Model file for the job. Use its own axes, mm. Coordinates: 2 decimals unless noted, no trailing zeros. Order: outer loops, then holes, each group sorted by start corner. A loop starts at its lowest first (then second) coordinate and runs counter-clockwise, first axis right, second up.
from build123d import *

# Parameters (mm, degrees)
SKETCH1_W           = 300
SKETCH1_H           = 400
SUPPORT_PLATE_DEPTH = 20
SKETCH2_R           = 6.5
BOLT_HOLES_DEPTH    = 21


with BuildPart() as part:
    # Sketch1 → Support Plate (new body)
    with BuildSketch(Plane(origin=(0, 0, 0), x_dir=(1, 0, 0), z_dir=(0, 1, 0))):
        Rectangle(SKETCH1_W, SKETCH1_H)
    extrude(amount=-SUPPORT_PLATE_DEPTH)

    # Sketch2 → Bolt Holes (cut, through all)
    with BuildSketch(Plane(origin=(0, 0, 0), x_dir=(-1, 0, 0), z_dir=(0, 1, 0))):
        with Locations((-100, -60)):
            Circle(SKETCH2_R)
        with Locations((50, -60)):
            Circle(SKETCH2_R)
        with Locations((50, 60)):
            Circle(SKETCH2_R)
        with Locations((-100, 60)):
            Circle(SKETCH2_R)
    extrude(amount=-BOLT_HOLES_DEPTH, mode=Mode.SUBTRACT)


solid = part.part
Q1. Probe line 1 (Z direction, x = -50, y = -7.75); line 2 (X direction, y = -9.25, z = 61.5); line 3 (Z direction, x = 97, y = -8.5). List the from-to ranges inside material, lowest first.
Established:
line 1: z = -200 to -66.5, -53.5 to 53.5, 66.5 to 200
line 2: x = -150 to -56.32, -43.68 to 93.68, 106.32 to 150
line 3: z = -200 to -65.77, -54.23 to 54.23, 65.77 to 200
Q2. Cut at A-A, the plane z = 60. List the corners of the cut face in (x, y), plus the area to 3 significant figures.
Established:
outline: (-150, -20) - (-56.5, -20) - (-56.5, 0) - (-150, 0) - close; (-43.5, -20) - (93.5, -20) - (93.5, 0) - (-43.5, 0) - close; (106.5, -20) - (150, -20) - (150, 0) - (106.5, 0) - close
area: 5,480 mm2
Q3. Cut at B-B, the plane x = -50. List the corners of the cut face in (y, z), plus the area to 3 significant figures.
Established:
outline: (-20, -200) - (0, -200) - (0, -66.5) - (-20, -66.5) - close; (-20, -53.5) - (0, -53.5) - (0, 53.5) - (-20, 53.5) - close; (-20, 66.5) - (0, 66.5) - (0, 200) - (-20, 200) - close
area: 7,480 mm2
Q4. Mould opens along Z. For faces 1 (the face through (-48.591, -9.86, 53.655)), 2 (the face through (-150, -10, 3)), 3 (the face through (-2, -10, -200)) say: pulls with the +Z half, pulls with the -Z half, needs draft (parallel to the pull), parting line crosses it, or undercut.
Established:
face 1: undercut
face 2: needs draft
face 3: pulls with the -Z half
